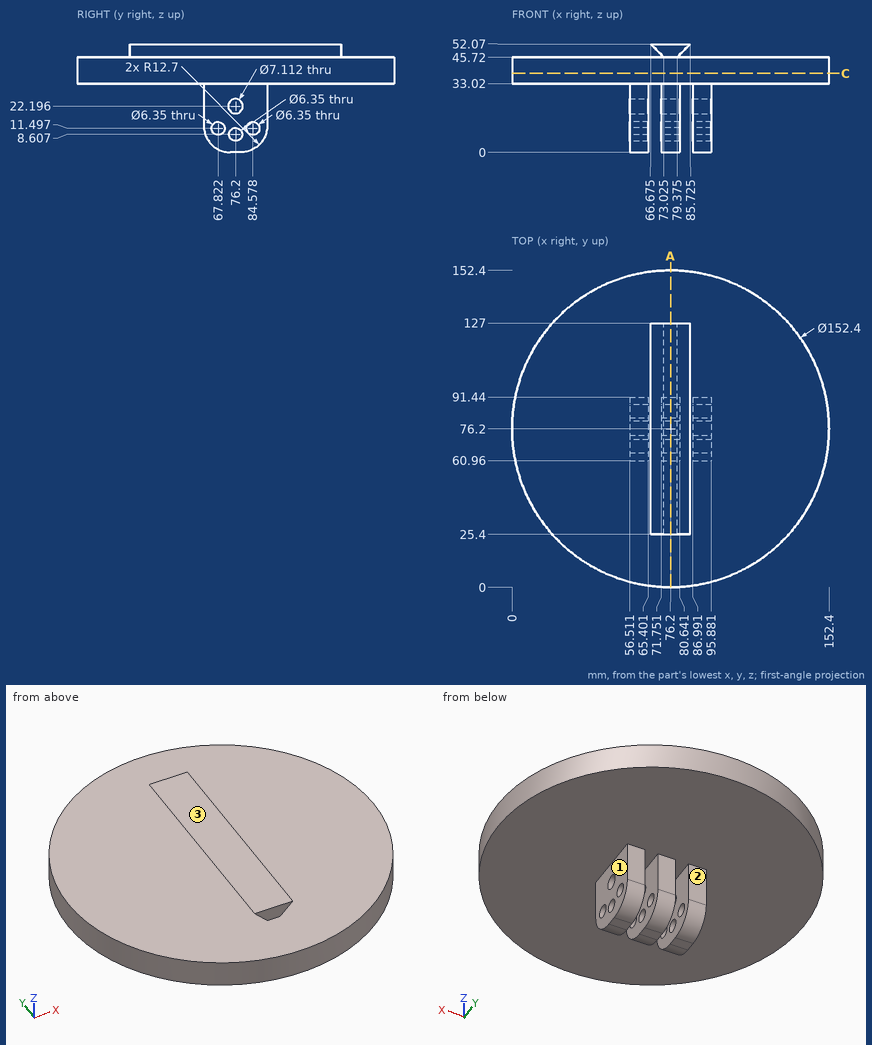
For this review, use the dimensioned drawing (mm, ordinates from the lowest corner) and the shaded views. A direction names the side the tool comes from. Give positions to 0.01 mm unless a question says otherwise; leave off trailing zeros. Write each loop counter-clockwise with the first axis right and the second up, starting at its lowest first coordinate (ties: lowest second). Pieces come first, ordered by that corner, then holes. Notation, with made-up numbers: M -1,-25.5 L 55,-25.5 A14 ccw 55,-17.5 Z; hole C -19.5,16 d9. An arc over 180 degrees is marked long. Answer as a JSON object with one key per item and string values. Group by question number.
Item 1: For pin 1 Ø4 at (x, y) = (122.5, 36.5) entering from -Z; pin 2 Ø5 at (y, z) = (84.58, 11.5) entering from +X; pin 3 Ø10 at (x, z) = (59.5, 22) entering from -Y; pin 4 Ø10 at (x, z) = (91, 25.5) entering from +Y, all flat-tipped, find the tip position at first contact; note any pin that passes through.
Item 2: Tool access review of the marked faces 1, 2 and 3: name each direction out of +Z, -Z, +X, -X, +Y, -Y from which nothing blocks a thin tool from reaching the whole face with its end or side.
Item 3: Consider section C-C on z = 38. Write out the cut boundary in (x, y).
Item 4: For probe 1 along Z at (x, y) = (119.5, 60); probe 2 along Y at (x, z) = (76, 21.5); probe 3 along Y at (x, z) = (64, 19), list the stretches that pass through material, from the lowest coordinate up. Write a range as [from, to].
Item 5: Consider section A-A on x = 76.2. Count the separate pieces of the cut face and the enclosed holes in it, plus the area to 3 significant figures.
Check result:
{
 "1": {"pin 1": "stops at z = 33.02", "pin 2": "passes through", "pin 3": "stops at y = 60.96", "pin 4": "stops at y = 91.44"},
 "2": {"face 1": "-Z, +X, +Y, -Y", "face 2": "-Z, +X, -X, +Y", "face 3": "+Z, +X, -X, +Y, -Y"},
 "3": {"outline": "C 76.2,76.2 d152.4"},
 "4": {"probe 1": "z = [33.02, 45.72]", "probe 2": "y = [60.96, 72.71], [79.69, 91.44]", "probe 3": "y = [60.96, 74.64], [77.76, 91.44]"},
 "5": {"separate pieces": "1", "enclosed holes": "4", "area": "3,380 mm^2"}
}
